Work out the finished part from the listing and answer in its coordinate system (mm). A direction names the side the tool comes from. Round coordinates to 2 decimals unless told otherwise and drop trailing zeros. Order: outer loops, then holes, each group sorted by start corner. A loop starts at its lowest first (then second) coordinate and runs counter-clockwise, first axis right, second up. Notation, with made-up numbers: M 74.5,-38.5 L 78.5,-38.5 A21 ccw 78.5,-19.5 Z; hole C 59.25,61.5 d10. An arc over 180 degrees is marked long. Answer as a JSON object with one key per item and string values. Group by question number.
from build123d import *

# Parameters (mm, degrees)
EXTRUDE_1_DEPTH     = 1.63
SKETCH_2_R          = 1.5
CUT_EXTRUDE_1_DEPTH = 36.99024208
SKETCH_8_W          = 51
SKETCH_8_H          = 5
EXTRUDE_6_DEPTH     = 3.68
SKETCH_9_W          = 7
SKETCH_9_H          = 2.7
EXTRUDE_7_DEPTH     = 3.5
SKETCH_10_W         = 7.53
SKETCH_10_H         = 5.24
EXTRUDE_8_DEPTH     = 2.66
SKETCH_11_W         = 22.18
SKETCH_11_H         = 21.945686578
EXTRUDE_9_DEPTH     = 2
SKETCH_12_W         = 6.42
SKETCH_12_H         = 6.42
EXTRUDE_10_DEPTH    = 1.5
SKETCH_13_W         = 3
SKETCH_13_H         = 3.86
EXTRUDE_11_DEPTH    = 1
SKETCH_14_R         = 3.84
EXTRUDE_12_DEPTH    = 5
SKETCH_15_W         = 3
SKETCH_15_H         = 1.5
EXTRUDE_13_DEPTH    = 0.64
EXTRUDE_14_DEPTH    = 0.6


with BuildPart() as part:
    # 草图1 → 凸台-拉伸1 (new body)
    with BuildSketch(Plane(origin=(0, 0, 0), x_dir=(1, 0, 0), z_dir=(0, 1, 0))):
        with BuildLine():
            Line((-29.5, 15.375), (29.5, 15.375))
            ThreePointArc((29.5, 15.375), (31.621320344, 14.496320344), (32.5, 12.375))
            Line((32.5, 12.375), (32.5, -12.375))
            ThreePointArc((32.5, -12.375), (31.621320344, -14.496320344), (29.5, -15.375))
            Line((29.5, -15.375), (-29.5, -15.375))
            ThreePointArc((-29.5, -15.375), (-31.621320344, -14.496320344), (-32.5, -12.375))
            Line((-32.5, -12.375), (-32.5, 12.375))
            ThreePointArc((-32.5, 12.375), (-31.621320344, 14.496320344), (-29.5, 15.375))
        make_face()
    extrude(amount=EXTRUDE_1_DEPTH)

    # 草图2 → 切除-拉伸1 (cut, through all)
    with BuildSketch(Plane(origin=(0, 1.63, 0), x_dir=(1, 0, 0), z_dir=(0, 1, 0))):
        with Locations(Location((-29, 11.875, 0), (0, 0, 270))):
            Circle(SKETCH_2_R)
        with Locations(Location((-29, -11.875, 0), (0, 0, 270))):
            Circle(SKETCH_2_R)
        with Locations(Location((29, -11.875, 0), (0, 0, 270))):
            Circle(SKETCH_2_R)
        with Locations(Location((29, 11.875, 0), (0, 0, 270))):
            Circle(SKETCH_2_R)
    extrude(amount=-CUT_EXTRUDE_1_DEPTH, mode=Mode.SUBTRACT)

    # 草图8 → 凸台-拉伸6 (add)
    with BuildSketch(Plane.XZ):
        with Locations((-0.2, -11.235)):
            Rectangle(SKETCH_8_W, SKETCH_8_H)
    extrude(amount=EXTRUDE_6_DEPTH)

    # 草图9 → 凸台-拉伸7 (add)
    with BuildSketch(Plane(origin=(0, 1.63, 0), x_dir=(1, 0, 0), z_dir=(0, 1, 0))):
        with Locations((-21.23, -14.025)):
            Rectangle(SKETCH_9_W, SKETCH_9_H)
    extrude(amount=EXTRUDE_7_DEPTH)

    # 草图10 → 凸台-拉伸8 (add)
    with BuildSketch(Plane(origin=(0, 1.63, 0), x_dir=(1, 0, 0), z_dir=(0, 1, 0))):
        with Locations((21.655, -12.755)):
            Rectangle(SKETCH_10_W, SKETCH_10_H)
    extrude(amount=EXTRUDE_8_DEPTH)

    # 草图11 → 凸台-拉伸9 (add)
    with BuildSketch(Plane(origin=(0, 1.63, 0), x_dir=(1, 0, 0), z_dir=(0, 1, 0))):
        with Locations((-4.38, 0.262156711)):
            Rectangle(SKETCH_11_W, SKETCH_11_H)
    extrude(amount=EXTRUDE_9_DEPTH)

    # 草图12 → 凸台-拉伸10 (add)
    with BuildSketch(Plane(origin=(0, 1.63, 0), x_dir=(1, 0, 0), z_dir=(0, 1, 0))):
        with Locations((-28.49, -3.575)):
            Rectangle(SKETCH_12_W, SKETCH_12_H)
    extrude(amount=EXTRUDE_10_DEPTH)

    # 草图13 → 凸台-拉伸11 (add)
    with BuildSketch(Plane(origin=(0, 1.63, 0), x_dir=(1, 0, 0), z_dir=(0, 1, 0))):
        with Locations((-28.52, 4.215)):
            Rectangle(SKETCH_13_W, SKETCH_13_H)
    extrude(amount=EXTRUDE_11_DEPTH)

    # 草图14 → 凸台-拉伸12 (add)
    with BuildSketch(Plane(origin=(0, 3.13, 0), x_dir=(1, 0, 0), z_dir=(0, 1, 0))):
        with Locations(Location((-28.49, -3.575, 0), (0, 0, 56.713583662))):
            Circle(SKETCH_14_R)
    extrude(amount=EXTRUDE_12_DEPTH)

    # 草图15 → 凸台-拉伸13 (add)
    with BuildSketch(Plane.XY.offset(15.375)):
        with Locations((-21.02, 3.38)):
            Rectangle(SKETCH_15_W, SKETCH_15_H)
    extrude(amount=EXTRUDE_13_DEPTH)

    # 草图16 → 凸台-拉伸14 (add)
    with BuildSketch(Plane.XY.offset(15.375)):
        Polygon((17.89, 3.79), (18.39, 4.29), (24.92, 4.29), (25.42, 3.79), (25.42, 2.63), (24.42, 1.63), (18.89, 1.63), (17.89, 2.63), align=None)
    extrude(amount=EXTRUDE_14_DEPTH)


solid = part.part
Item 1: Consider L1, parallel to X at y = 3.25, z = 14; L2, parallel to Z at x = -7.5, y = -1.5 (3 decimals); L3, parallel to Y at x = 14, z = -7.5. Determine where each line is inside the solid, lowest interval first.
Item 2: A tool of negligible diameter and unlimited length cuts with its end or side. For faces 1 (the flat face through (-29, 2, 6.785)), 2 (the flat face through (-31.4, 3.13, 6.5)), 3 (the flat face through (-1, -2, -8.735)), from which of +Z, -Z, +X, -X, +Y, -Y can it reach the whole face along a straight path? Write none if from no direction.
Item 3: The mould has two halves that part along X. Classify faces 4 (the cylindrical face through (31.645, 0.804, 14.473)), 5 (the flat face through (-25.6, 3.13, 0.7)), 6 (the flat face through (-21, 3, 12.675)): +X half, -X half, draft (parallel to the pull), parting line (faces both ways), or undercut.
Item 4: Find section B-B (x = 16). Give the vertices of the cut face in (y, z) (3 decimals).
Item 5: Each of these flat-tipped pins is pushed along its axis until it touches: pin 1 (9 mm diameter, centred on x = -6, z = 4, fed in from +Y); pin 2 (1.5 mm diameter, centred on x = 18.5, z = -6, fed in from -Y); pin 3 (3 mm diameter, centred on y = 2.5, z = 14.5, fed in from -X); pin 4 (3 mm diameter, centred on x = 5, y = -1, fed in from -Z) (3 decimals). Where does it stop, or does it pass through?
Item 6: Find section A-A (z = -3). Give the vertices of the cut face in (x, y), and give its area (3 significant figures).
Item 7: Find section D-D (x = -10). Give the vertices of the cut face in (y, z) (3 decimals).
Item 8: Find section C-C (y = -1). Give the vertices of the cut face in (x, z) (3 decimals).
Responses:
{
 "1": {"L1": "x = -24.73 to -17.73, 17.89 to 25.42", "L2": "z = -13.735 to -8.735", "L3": "y = 0 to 1.63"},
 "2": {"face 1": "+Z, -X", "face 2": "+Z, -X, +Y", "face 3": "+Z, +X, -X, -Y"},
 "3": {"face 4": "+X half", "face 5": "undercut", "face 6": "draft"},
 "4": {"outline": "M -3.68,-13.735 L 0,-13.735 L 0,-15.375 L 1.63,-15.375 L 1.63,15.375 L 0,15.375 L 0,-8.735 L -3.68,-8.735 Z"},
 "5": {"pin 1": "stops at y = 3.63", "pin 2": "stops at y = 0", "pin 3": "stops at x = -32.36", "pin 4": "stops at z = -15.375"},
 "6": {"outline": "M -32.5,0 L 32.5,0 L 32.5,1.63 L 6.71,1.63 L 6.71,3.63 L -15.47,3.63 L -15.47,1.63 L -27.02,1.63 L -27.02,2.63 L -30.02,2.63 L -30.02,1.63 L -32.5,1.63 Z", "area": "153 mm^2"},
 "7": {"outline": "M -3.68,-13.735 L 0,-13.735 L 0,-15.375 L 1.63,-15.375 L 1.63,-11.235 L 3.63,-11.235 L 3.63,10.711 L 1.63,10.711 L 1.63,15.375 L 0,15.375 L 0,-8.735 L -3.68,-8.735 Z"},
 "8": {"outline": "M -25.7,-13.735 L 25.3,-13.735 L 25.3,-8.735 L -25.7,-8.735 Z"}
}
